Autodesk Inventor part; units mm, degrees
ref_plane "YZ Plane" through (0, 0, 0) normal (1, 0, 0) x (0, 1, 0)
ref_plane "XZ Plane" through (0, 0, 0) normal (0, 1, 0) x (-1, 0, 0)
ref_plane "XY Plane" through (0, 0, 0) normal (0, 0, 1) x (1, 0, 0)
sketch "Profile" plane through (0, 0, 0) normal (0, 0, 1) x (1, 0, 0)
  line L0 (-21.6, 0) -> (-21.6, 11)
  line L1 (-21.6, 11) -> (0, 11)
  line L2 (0, 11) -> (0.5774, 12)
  line L3 (0.5774, 12) -> (45.5774, 12)
  line L4 (45.5774, 12) -> (46.1547, 11)
  line L5 (46.1547, 11) -> (68.4, 11)
  line L6 (68.4, 11) -> (68.4, 0)
  line L7 (-21.6, 0) -> (0, 0)
  line L8 (0, 0) -> (0, 9)
  line L9 (0, 9) -> (60.4, 9)
  line L10 (60.4, 9) -> (60.4, 0)
  line L11 (60.4, 0) -> (68.4, 0)
  line L12 (-39.6, 0) -> (86.4, 0) construction
  line L13 (0, 11) -> (0, 9) construction
  dimension "BodyLength" = 90
  dimension "d1" = 11
  dimension "d3" = 120
  dimension "d4" = 120
  dimension "d5" = 45
  dimension "d6" = 21.6
  dimension "d16" = 8
  dimension "d29" = 1
  dimension "d30" = 9
revolve "ProfileRevolveFeature" add sketch "Profile" angle 360 about axis through (-10, 0, 0) along (1, 0, 0)
sketch "InsideHole" plane through (-21.6, 0, 0) normal (-1, 0, 0) x (0, 0, 1)
  circle A0 centre (0, 0) radius 9 construction
hole "InsideHoleFeature" at (-21.6, 0, 0) direction (1, 0, 0) diameter 19 end through all
chamfer "EndChamferFeature" distance 1 angle 45 1 edges at (-21.6, -11, 0)
sketch "CapMountHole" plane through (0, 0, 0) normal (0, 1, 0) x (-1, 0, 0)
  line L0 (-68.4, 11) -> (-68.4, -11) construction
  line L1 (10.64, 0) -> (-63.84, 0) construction
  circle A0 centre (-63.9, 0) radius 1.25
  point P0 (0, 0)
  dimension "d31" = 4.5
  dimension "d39" = 2.5
extrude "CapMountHoleFeature" cut sketch "CapMountHole" along normal through all both and the other way through all
equation "\"d5\" = 0.5 * BodyLength"
equation "\"d6\" = 0.24 * BodyLength"
properties part number "BackPair1PistonBody"
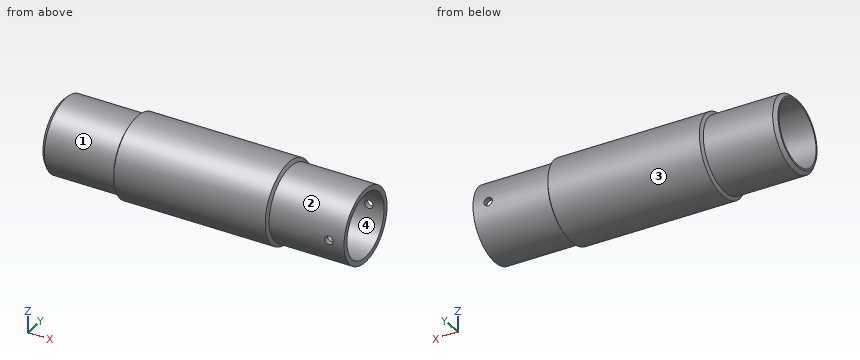
Build history of the part. All positions in model axes, mm. Face numbers are marked on the shaded views. A direction names the side the tool comes from. Coordinates: 2 decimals unless noted, no trailing zeros. Order: outer loops, then holes, each group sorted by start corner. A loop starts at its lowest first (then second) coordinate and runs counter-clockwise, first axis right, second up. Notation, with made-up numbers: (-8.5, 69.25) - (50.5, 69.25) arc R21 cw to (50.5, 101.25) - close; hole circle Ø5 at (-38, 87.25). An arc over 180 degrees is marked (long way). Write each question's results on one line, items separated by ' | '. Start each with the question number.
Item 1: Band-saw the part on B-B on z = 0. Write the cut outline in (x, y), and give its area (3 significant figures).
Item 2: Wall check: probe 1 along Z at (x, y) = (19, 0); probe 2 along X at (y, z) = (10, 0); probe 3 along X at (y, z) = (10.2, 0). Give the ranges that are in metal, low to high. Write a range as [from, to].
Item 3: Band-saw the part on D-D on x = 28. Write the cut outline in (y, z).
Item 4: Tool access for the marked faces 1 and 2: list every direction of +Z, -Z, +X, -X, +Y, -Y with a clear straight run to the whole face (end or side of a thin tool).
Item 5: Band-saw the part on C-C on x = 63.9. Write the cut outline in (y, z), and give its area (3 significant figures).
Item 6: Mould opens along Y. For the marked faces 3 and 4 say: released by +Y, released by -Y, zero draft, split by the parting line, or undercut.
Item 7: Band-saw the part on A-A on y = 0. Write the cut outline in (x, z), and give its area (3 significant figures).
Item 8: Flat gauge pins, fed straight in: pin 1 (8 mm diameter, centred on x = 19.5, z = -6.5, fed in from +Y); pin 2 (1 mm diameter, centred on x = 29.5, z = -1, fed in from -Y); pin 3 (5 mm diameter, centred on x = 53.5, y = -3.5, fed in from -Z); pin 4 (1.5 mm diameter, centred on x = 63.9, z = 0, fed in from -Y). Where does each tip first touch, or does it go through?
Numbers:
1) outline: (-21.6, -10) - (-20.6, -11) - (0, -11) - (0.58, -12) - (45.58, -12) - (46.15, -11) - (62.65, -11) - (62.65, -9.5) - (-21.6, -9.5) - close; (-21.6, 9.5) - (62.65, 9.5) - (62.65, 11) - (46.15, 11) - (45.58, 12) - (0.58, 12) - (0, 11) - (-20.6, 11) - (-21.6, 10) - close; (65.15, -11) - (68.4, -11) - (68.4, -9.5) - (65.15, -9.5) - close; (65.15, 9.5) - (68.4, 9.5) - (68.4, 11) - (65.15, 11) - close | area: 353 mm^2
2) probe 1: [-12, -9.5], [9.5, 12] | probe 2: [-21.6, 62.65], [65.15, 68.4] | probe 3: [-21.4, 62.65], [65.15, 68.4]
3) outline: circle Ø24 at (0, 0); hole circle Ø19 at (0, 0)
4) face 1: -X | face 2: +X
5) outline: (-10.93, -1.25) arc R11 ccw to (10.93, -1.25) - (9.42, -1.25) arc R9.5 cw to (-9.42, -1.25) - close; (-10.93, 1.25) - (-9.42, 1.25) arc R9.5 cw to (9.42, 1.25) - (10.93, 1.25) arc R11 ccw to start | area: 89.1 mm^2
6) face 3: split by the parting line | face 4: undercut
7) outline: (-21.6, -10) - (-20.6, -11) - (0, -11) - (0.58, -12) - (45.58, -12) - (46.15, -11) - (68.4, -11) - (68.4, -9.5) - (-21.6, -9.5) - close; (-21.6, 9.5) - (68.4, 9.5) - (68.4, 11) - (46.15, 11) - (45.58, 12) - (0.58, 12) - (0, 11) - (-20.6, 11) - (-21.6, 10) - close | area: 360 mm^2
8) pin 1: y = 11.74 | pin 2: y = -11.99 | pin 3: z = -10.95 | pin 4: through
